from build123d import *

# Parameters (mm, degrees)
CROQUIS1_R              = 2.1
SALIENTE_EXTRUIR1_DEPTH = 2
CROQUIS2_W              = 20
CROQUIS2_H              = 2
SALIENTE_EXTRUIR2_DEPTH = 8
CROQUIS3_R              = 3.5
CROQUIS3_R_2            = 2.1
SALIENTE_EXTRUIR3_DEPTH = 2


with BuildPart() as part:
    # Croquis1 → Saliente-Extruir1 (new body)
    with BuildSketch(Plane(origin=(0, 0, 0), x_dir=(1, 0, 0), z_dir=(0, 1, 0))):
        with BuildLine():
            Line((-21, 4.25), (21, 4.25))
            ThreePointArc((21, 4.25), (23.870499774, 3.134123649), (25.233647636, 0.372461669))
            Line((25.233647636, 0.372461669), (31.233647636, -67.827538331))
            ThreePointArc((31.233647636, -67.827538331), (30.134123649, -71.070499774), (27, -72.45))
            Line((27, -72.45), (-27, -72.45))
            ThreePointArc((-27, -72.45), (-30.134123649, -71.070499774), (-31.233647636, -67.827538331))
            Line((-31.233647636, -67.827538331), (-25.233647636, 0.372461669))
            ThreePointArc((-25.233647636, 0.372461669), (-23.870499774, 3.134123649), (-21, 4.25))
        make_face()
        with Locations(Location((-21, 0, 0), (0, 0, 270))):
            Circle(CROQUIS1_R, mode=Mode.SUBTRACT)
        with Locations(Location((21, 0, 0), (0, 0, 90))):
            Circle(CROQUIS1_R, mode=Mode.SUBTRACT)
        with Locations(Location((0, -30.2, 0), (0, 0, 270))):
            Circle(CROQUIS1_R, mode=Mode.SUBTRACT)
        with Locations(Location((-27, -68.2, 0), (0, 0, 270))):
            Circle(CROQUIS1_R, mode=Mode.SUBTRACT)
        with Locations(Location((27, -68.2, 0), (0, 0, 270))):
            Circle(CROQUIS1_R, mode=Mode.SUBTRACT)
        with Locations(Location((-15, -37.2, 0), (0, 0, 270))):
            Circle(CROQUIS1_R, mode=Mode.SUBTRACT)
        with Locations(Location((-15, -57.2, 0), (0, 0, 270))):
            Circle(CROQUIS1_R, mode=Mode.SUBTRACT)
        with Locations(Location((15, -37.2, 0), (0, 0, 270))):
            Circle(CROQUIS1_R, mode=Mode.SUBTRACT)
        with BuildLine():
            Line((9.8, -52.2), (23.8, -52.2))
            ThreePointArc((23.8, -52.2), (25.8, -54.2), (23.8, -56.2))
            Line((23.8, -56.2), (9.8, -56.2))
            ThreePointArc((9.8, -56.2), (7.8, -54.2), (9.8, -52.2))
        make_face(mode=Mode.SUBTRACT)
    extrude(amount=SALIENTE_EXTRUIR1_DEPTH)

    # Croquis2 → Saliente-Extruir2 (add)
    with BuildSketch(Plane(origin=(0, 2, 0), x_dir=(1, 0, 0), z_dir=(0, 1, 0))):
        with Locations((0, -3.25)):
            Rectangle(CROQUIS2_W, CROQUIS2_H)
        with Locations((0, 3.25)):
            Rectangle(CROQUIS2_W, CROQUIS2_H)
    extrude(amount=SALIENTE_EXTRUIR2_DEPTH)

    # Croquis3 → Saliente-Extruir3 (add)
    # profile 1 of 5: a face of its own
    with BuildSketch(Plane(origin=(0, 2, 0), x_dir=(1, 0, 0), z_dir=(0, 1, 0))):
        with Locations(Location((15, -37.2, 0), (0, 0, 270))):
            Circle(CROQUIS3_R)
        with Locations(Location((15, -37.2, 0), (0, 0, 270))):
            Circle(CROQUIS3_R_2, mode=Mode.SUBTRACT)
    # profile 2 of 5: a face of its own
    with BuildSketch(Plane(origin=(0, 2, 0), x_dir=(1, 0, 0), z_dir=(0, 1, 0))):
        with Locations(Location((-15, -37.2, 0), (0, 0, 270))):
            Circle(CROQUIS3_R)
        with Locations(Location((-15, -37.2, 0), (0, 0, 270))):
            Circle(CROQUIS3_R_2, mode=Mode.SUBTRACT)
    # profile 3 of 5: a face of its own
    with BuildSketch(Plane(origin=(0, 2, 0), x_dir=(1, 0, 0), z_dir=(0, 1, 0))):
        with Locations(Location((-15, -57.2, 0), (0, 0, 270))):
            Circle(CROQUIS3_R)
        with Locations(Location((-15, -57.2, 0), (0, 0, 270))):
            Circle(CROQUIS3_R_2, mode=Mode.SUBTRACT)
    # profile 4 of 5: a face of its own
    with BuildSketch(Plane(origin=(0, 2, 0), x_dir=(1, 0, 0), z_dir=(0, 1, 0))):
        with BuildLine():
            Line((-25.5, -44.25), (-25.5, -49.25))
            ThreePointArc((-25.5, -49.25), (-24, -50.75), (-22.5, -49.25))
            Line((-22.5, -49.25), (-22.5, -44.25))
            ThreePointArc((-22.5, -44.25), (-24, -42.75), (-25.5, -44.25))
        make_face()
    # profile 5 of 5: a face of its own
    with BuildSketch(Plane(origin=(0, 2, 0), x_dir=(1, 0, 0), z_dir=(0, 1, 0))):
        with BuildLine():
            Line((22.5, -44.25), (22.5, -49.25))
            ThreePointArc((22.5, -49.25), (24, -50.75), (25.5, -49.25))
            Line((25.5, -49.25), (25.5, -44.25))
            ThreePointArc((25.5, -44.25), (24, -42.75), (22.5, -44.25))
        make_face()
    extrude(amount=SALIENTE_EXTRUIR3_DEPTH)


solid = part.part
Here's how the part is built. I have some questions about the finished solid (model axes, mm). A direction names the side the tool comes from. Round coordinates to 2 decimals unless told otherwise and drop trailing zeros. Loops run counter-clockwise (first coordinate to the right, second up) from the corner with the lowest first, then second, coordinate; pieces in that order, holes last.
1. We'd pull the mould along Z, two halves only. Please class faces 1 (the face through (0, 1, 72.45)), 2 (the face through (10, 6, 3)), 3 (the face through (0, 4, -4.25)), 4 (the face through (-16.341, 2.986, 60.433)): +Z half, -Z half, draft (parallel to the pull), parting line (faces both ways), or undercut.
Answer list:
face 1: +Z half
face 2: draft
face 3: -Z half
face 4: undercut
2. For P1, Ø2, axis at x = 3, z = 63.5, coming from the +Y side; P2, Ø0.6, axis at y = 3, z = 46, coming from the -X side; P3, Ø0.6, axis at y = 6, z = 3.5, coming from the +X side, each with a flat end and sliding along its axis, tell me the tip position at first contact or that it passes through.
Answer list:
P1: stops at y = 2
P2: stops at x = -25.5
P3: stops at x = 10
3. If we section it at A-A on y = 8.5: Write out the boundary of the cut face in (x, z).
Answer list:
outline: (-10, -4.25) - (10, -4.25) - (10, -2.25) - (-10, -2.25) - close; (-10, 2.25) - (10, 2.25) - (10, 4.25) - (-10, 4.25) - close
4. Which directions (+Z, -Z, +X, -X, +Y, -Y) give clear straight access to the entire face, cutting with the end or side of a thin tool? Please do faces 5 (the face through (10, 6, -3)), 6 (the face through (22.5, 3, 47)), 7 (the face through (-23.97, 2.99, 42.75)), 8 (the face through (-24.03, 2.99, 50.75)), 9 (the face through (25.8, 1, 54.2)).
Answer list:
face 5: +Z, -Z, +X, +Y
face 6: +Z, -Z, +Y
face 7: -Z, +Y
face 8: +Z, +Y
face 9: +Y, -Y
5. If we section it at C-C on z = 24: Write out the boundary of the cut face in (x, y), plus the area to 3 significant figures.
Answer list:
outline: (-27.38, 0) - (27.38, 0) - (27.38, 2) - (-27.38, 2) - close
area: 110 mm2
6. If we section it at B-B on x = 14: Write out the boundary of the cut face in (y, z).
Answer list:
outline: (0, -4.25) - (2, -4.25) - (2, 33.85) - (4, 33.85) - (4, 35.35) - (0, 35.35) - close; (0, 39.05) - (4, 39.05) - (4, 40.55) - (2, 40.55) - (2, 52.2) - (0, 52.2) - close; (0, 56.2) - (2, 56.2) - (2, 72.45) - (0, 72.45) - close
7. If I drill on line 1 along X through (y, z) = (2.3, 37.2); line 2 along Z through (x, y) = (5, 9.75); line 3 along X through (y, z) = (3, 57.2), over which ranges is the centre line in solid material (lowest first)?
Answer list:
line 1: x = -18.5 to -17.1, -12.9 to -11.5, 11.5 to 12.9, 17.1 to 18.5
line 2: z = -4.25 to -2.25, 2.25 to 4.25
line 3: x = -18.5 to -17.1, -12.9 to -11.5
8. If we section it at D-D on z = 15: Write out the boundary of the cut face in (x, y).
Answer list:
outline: (-26.59, 0) - (26.59, 0) - (26.59, 2) - (-26.59, 2) - close
